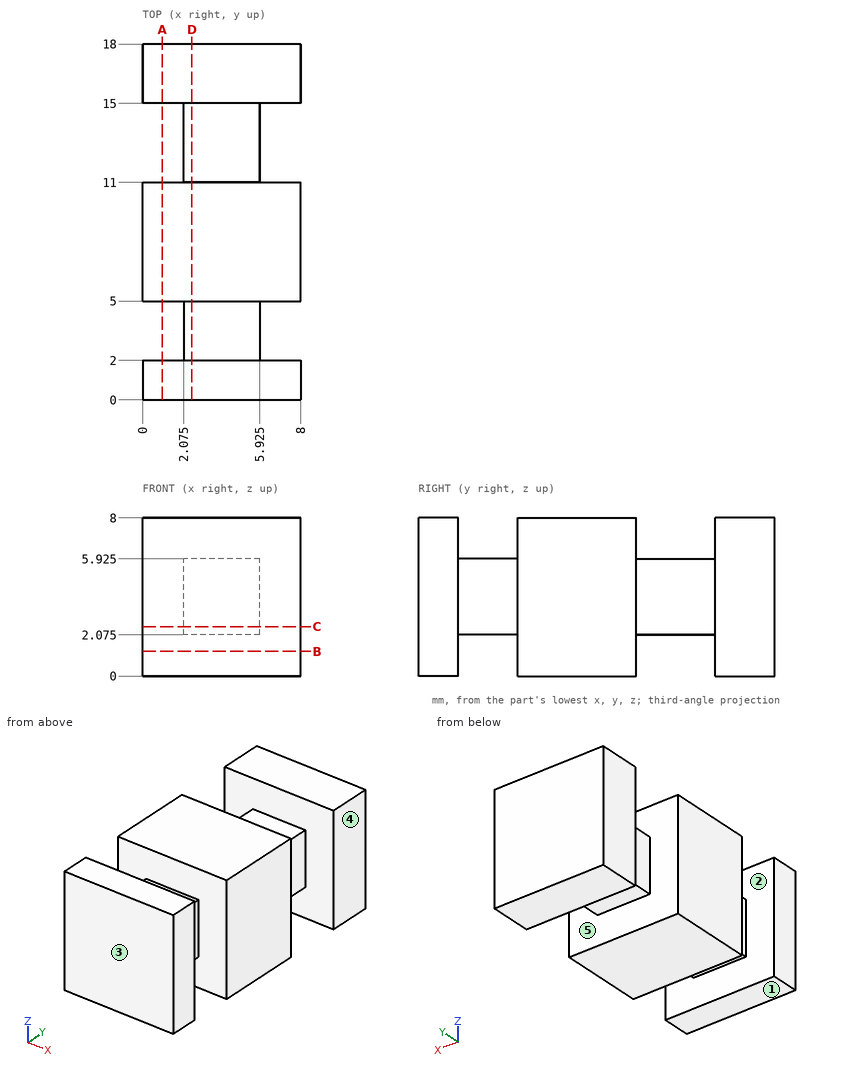
Input: dimensioned drawing with shaded views. Units: mm. Origin: part minimum x, y, z. A direction names the side the tool comes from. Give positions to 0.01 mm unless a question says otherwise; leave off trailing zeros. Write each loop counter-clockwise with the first axis right and the second up, starting at its lowest first coordinate (ties: lowest second). Pieces come first, ordered by that corner, then holes. Notation, with made-up numbers: (-16, 76.5) - (21, 76.5) arc R8 ccw to (21, 87.5) - close; hole circle Ø8 at (-14.75, -1.75). An arc over 180 degrees is marked (long way). Write item = value, one per line. Start each with the question number.
1) Cut plane C-C (z = 2.5). Return loops of the section in (x, y) (3 decimals), and give its area (3 significant figures).
2) Material intervals for L1, parallel to Y at x = 4.5, z = 1; L2, parallel to Z at x = 3.75, y = 11.5 (3 decimals), sorted ascending. Write a range as [from, to].
3) Pin query (flat end, axial travel): pin 1 (1.5 mm diameter, centred on y = 15.5, z = 4.5, fed in from -X); pin 2 (1.2 mm diameter, centred on x = 4, y = 13.5, fed in from +Z) (3 decimals); pin 3 (0.9 mm diameter, centred on y = 4, z = 3, fed in from +X) (3 decimals); pin 4 (1.2 mm diameter, centred on x = 4, y = 13, fed in from -Z) (3 decimals). Return the tip coordinate at first contact, or that it passes through.
4) Cut plane D-D (x = 2.5). Return loops of the section in (y, z) (3 decimals).
5) Cut plane A-A (x = 1). Return loops of the section in (y, z), and give its area (3 significant figures).
6) Cut plane B-B (z = 1.25). Return loops of the section in (x, y), and give its area (3 significant figures).
7) Draft query along Y for the marked faces 1, 2 and 3. Return one class per face: pulls with the +Y half, pulls with the -Y half, needs draft (parallel to the pull), parting line crosses it, or undercut.
8) Reachability of the marked faces 4 and 5 from +Z, -Z, +X, -X, +Y, -Y: full face, straight path, thin tool, end or side. Return the list, or none.
Answers follow:
q1.outline = (0, 0) - (8, 0) - (8, 2) - (5.925, 2) - (5.925, 5) - (8, 5) - (8, 11) - (5.925, 11) - (5.925, 15) - (8, 15) - (8, 18) - (0, 18) - (0, 15) - (2.075, 15) - (2.075, 11) - (0, 11) - (0, 5) - (2.075, 5) - (2.075, 2) - (0, 2) - close
q1.area = 115 mm^2
q2.L1 = [0, 2], [5, 11], [15, 18]
q2.L2 = [2.075, 5.925]
q3.pin_1 = 0
q3.pin_2 = 5.925
q3.pin_3 = 5.925
q3.pin_4 = 2.075
q4.outline = (0, 0) - (2, 0) - (2, 2.075) - (5, 2.075) - (5, 0) - (11, 0) - (11, 2.075) - (15, 2.075) - (15, 0) - (18, 0) - (18, 8) - (15, 8) - (15, 5.925) - (11, 5.925) - (11, 8) - (5, 8) - (5, 5.925) - (2, 5.925) - (2, 8) - (0, 8) - close
q5.outline = (0, 0) - (2, 0) - (2, 8) - (0, 8) - close; (5, 0) - (11, 0) - (11, 8) - (5, 8) - close; (15, 0) - (18, 0) - (18, 8) - (15, 8) - close
q5.area = 88.0 mm^2
q6.outline = (0, 0) - (8, 0) - (8, 2) - (0, 2) - close; (0, 5) - (8, 5) - (8, 11) - (0, 11) - close; (0, 15) - (8, 15) - (8, 18) - (0, 18) - close
q6.area = 88.0 mm^2
q7.face_1 = needs draft
q7.face_2 = undercut
q7.face_3 = pulls with the -Y half
q8.face_4 = +Z, -Z, +X, +Y, -Y
q8.face_5 = none
